from build123d import *

# Parameters (mm, degrees)
SKETCH1_R           = 9.9
BOSS_EXTRUDE1_DEPTH = 9
SKETCH2_R           = 12
BOSS_EXTRUDE2_DEPTH = 6
SKETCH3_R           = 9.9
BOSS_EXTRUDE3_DEPTH = 7
SKETCH7_R           = 15
SKETCH7_R_2         = 12
CUT_EXTRUDE3_DEPTH  = 1
SKETCH10_R          = 1.5
CUT_EXTRUDE4_DEPTH  = 23
SKETCH12_R          = 1.5
CUT_EXTRUDE5_DEPTH  = 12
CHAMFER1_SIZE       = 1


with BuildPart() as part:
    # Sketch1 → Boss-Extrude1 (new body)
    with BuildSketch(Plane(origin=(0, 0, 0), x_dir=(1, 0, 0), z_dir=(0, 1, 0))):
        Circle(SKETCH1_R)
    extrude(amount=BOSS_EXTRUDE1_DEPTH)

    # Sketch2 → Boss-Extrude2 (add)
    with BuildSketch(Plane(origin=(0, 9, 0), x_dir=(1, 0, 0), z_dir=(0, 1, 0))):
        Circle(SKETCH2_R)
    extrude(amount=BOSS_EXTRUDE2_DEPTH)

    # Sketch3 → Boss-Extrude3 (add)
    with BuildSketch(Plane(origin=(0, 15, 0), x_dir=(1, 0, 0), z_dir=(0, 1, 0))):
        with Locations((0, 2.5)):
            Circle(SKETCH3_R)
    extrude(amount=BOSS_EXTRUDE3_DEPTH)

    # Sketch7 → Cut-Extrude3 (cut)
    with BuildSketch(Plane(origin=(0, 15, 0), x_dir=(1, 0, 0), z_dir=(0, 1, 0))):
        with Locations((0, 2.5)):
            Circle(SKETCH7_R)
        with Locations((0, 2.5)):
            Circle(SKETCH7_R_2, mode=Mode.SUBTRACT)
    extrude(amount=-CUT_EXTRUDE3_DEPTH, mode=Mode.SUBTRACT)

    # Sketch10 → Cut-Extrude4 (cut, through all)
    with BuildSketch(Plane(origin=(0, 22, 0), x_dir=(1, 0, 0), z_dir=(0, 1, 0))):
        with Locations((5.5, 0)):
            Circle(SKETCH10_R)
        with Locations((-5.5, 0)):
            Circle(SKETCH10_R)
    extrude(amount=-CUT_EXTRUDE4_DEPTH, mode=Mode.SUBTRACT)

    # Sketch12 → Cut-Extrude5 (cut)
    with BuildSketch(Plane(origin=(0, 0, 0), x_dir=(-1, 0, 0), z_dir=(0, -1, 0))):
        with Locations((0, 5.5)):
            Circle(SKETCH12_R)
        with Locations((0, -5.5)):
            Circle(SKETCH12_R)
    extrude(amount=-CUT_EXTRUDE5_DEPTH, mode=Mode.SUBTRACT)

    # Chamfer1
    chamfer1_edges = [part.edges().sort_by_distance(p)[0] for p in [
        (-9.9, 22, -2.5),
        (-9.9, 0, 0),
    ]]
    chamfer(chamfer1_edges, length=CHAMFER1_SIZE)


solid = part.part
Verification items for the finished model (mm, model axes). A direction names the side the tool comes from. Coordinates: 2 decimals unless noted, no trailing zeros. Order: outer loops, then holes, each group sorted by start corner. A loop starts at its lowest first (then second) coordinate and runs counter-clockwise, first axis right, second up. Notation, with made-up numbers: (81, 76) -> (121, 76) arc R21 cw to (121, 112) -> close; hole circle Ø4 at (-1, 84). An arc over 180 degrees is marked (long way). Use CSV: the item, a comma, the result in double quotes. Start each with the question number.
Q1. Section check C-C, the plane y = 19.75. Record the cut outline in (x, z).
Q2. Section check D-D, the plane z = 0.5. Give the number of separate pieces and of enclosed holes in the cut face, and give its area (3 significant figures).
Q3. Thickness scan on line 1 along X through (y, z) = (12.75, 0); line 2 along Z through (x, y) = (0, 5.25); line 3 along X through (y, z) = (21, 0.75). Record the ranges inside material, lowest first.
Q4. Section check A-A, the plane y = 4.5. Record the cut outline in (x, z), and give its area (3 significant figures).
Q5. Section check B-B, the plane x = 0. Record the cut outline in (y, z), and give its area (3 significant figures).
Q6. Depth check by flat-ended pin: P1, Ø2.5, axis at x = 0, z = -5.5, coming from the -Y side; P2, Ø1, axis at x = 1.5, z = -11.5, coming from the -Y side; P3, Ø5, axis at y = 18, z = 4.5, coming from the -X side. Enter the tip coordinate at first touch or a pass-through.
Q7. Tool access check on faces 1 (the cylindrical face through (-2.146, 17.958, 7.165)), 2 (the cylindrical face through (4.3, 11.2, 0.9)), 3 (the cylindrical face through (-0.2, 14.5, 9.5)), 4 (the flat face through (0, 12, 5)). Record the directions out of +Z, -Z, +X, -X, +Y, -Y that give a thin tool (end or side, any length) a straight path to the whole face; none if there is none.
Q8. Draft check along Z on faces 5 (the cylindrical face through (9.443, 4.944, -2.974)), 6 (the cylindrical face through (-6.7, 11.2, 0.9)), 7 (the flat face through (0, 0, 0)). Enter one of: +Z half, -Z half, draft (parallel to the pull), parting line (faces both ways), or undercut.
Returned:
1,outline,"circle Ø19.8 at (0, -2.5); hole circle Ø3 at (-5.5, 0); hole circle Ø3 at (5.5, 0)"
2,separate pieces,"3"
2,enclosed holes,"0"
2,area,"327 mm^2"
3,line 1,"x = -12 to -7, -4 to 4, 7 to 12"
3,line 2,"z = -9.9 to -7, -4 to 4, 7 to 9.9"
3,line 3,"x = -9.35 to -6.8, -4.2 to 4.2, 6.8 to 9.35"
4,outline,"circle Ø19.8 at (0, 0); hole circle Ø3 at (-5.5, 0); hole circle Ø3 at (0, -5.5); hole circle Ø3 at (0, 5.5); hole circle Ø3 at (5.5, 0)"
4,area,"280 mm^2"
5,outline,"(0, -8.9) -> (1, -9.9) -> (9, -9.9) -> (9, -12) -> (15, -12) -> (15, -12.4) -> (21, -12.4) -> (22, -11.4) -> (22, 6.4) -> (21, 7.4) -> (15, 7.4) -> (15, 9.5) -> (14, 9.5) -> (14, 12) -> (9, 12) -> (9, 9.9) -> (1, 9.9) -> (0, 8.9) -> (0, 7) -> (12, 7) -> (12, 4) -> (0, 4) -> (0, -4) -> (12, -4) -> (12, -7) -> (0, -7) -> close"
5,area,"384 mm^2"
6,P1,"stops at y = 12"
6,P2,"stops at y = 9"
6,P3,"stops at x = -8.82"
7,face 1,"+Y"
7,face 2,"+Y, -Y"
7,face 3,"+Z, +Y"
7,face 4,"-Y"
8,face 5,"parting line"
8,face 6,"undercut"
8,face 7,"draft"
